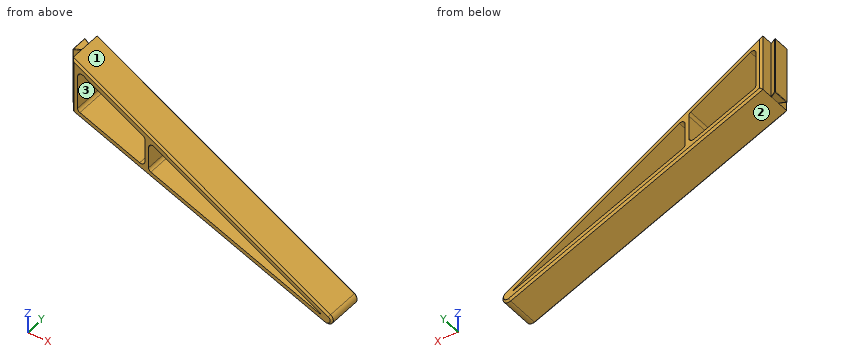
```python
from build123d import *

# Parameters (mm, degrees)
F1_DEPTH = 20
F3_DEPTH = 30
F4_R     = 2
F5_SIZE  = 1
F6_R     = 0.25


with BuildPart() as f1:
    # F0 (on Front) → F1 (new body)
    with BuildSketch(Plane.XZ):
        with BuildLine():
            Line((-46, 30), (-46, 0))
            Line((-46, 0), (89.051266, -55.940066))
            ThreePointArc((89.051266, -55.940066), (92.886071, -54.503098), (91.714375, -50.579104))
            Line((91.714375, -50.579104), (-46, 30))
        make_face()
        Polygon((-5, 2.534367), (90.199316, -53.168427), (-5, -13.735579), (-7, -12.907152), (-43, 2.004536), (-43, 24.768836), (-7, 3.704603), align=None, mode=Mode.SUBTRACT)
        Polygon((-5, -13.735579), (-5, 2.534367), (-7, 3.704603), (-7, -12.907152), align=None)
    extrude(amount=F1_DEPTH)

    # F2 (on Top) → F3 (join)
    with BuildSketch(Plane.XY):
        Polygon((-49.464102, -14.75), (-46, -12.75), (-46, -7.25), (-49.464102, -5.25), align=None)
    extrude(amount=F3_DEPTH)

    # F4
    f4_edges = [f1.edges().sort_by_distance(p)[0] for p in [
        (-7, -10, -12.907152),
        (-43, -10, 2.004536),
        (-43, -10, 24.768836),
        (-7, -10, 3.704603),
        (-5, -10, 2.534367),
        (-5, -10, -13.735579),
    ]]
    fillet(f4_edges, radius=F4_R)

    # F5
    f5_edges = [f1.edges().sort_by_distance(p)[0] for p in [
        (-46, 0, 15),
        (-46, -20, 15),
        (21.525633, -20, -27.970033),
        (21.525633, 0, -27.970033),
    ]]
    chamfer(f5_edges, length=F5_SIZE)

    # F6
    f6_edges = [f1.edges().sort_by_distance(p)[0] for p in [
        (-49.464102, -14.75, 15),
        (-49.464102, -5.25, 15),
        (-49.464102, -10, 0),
        (-49.464102, -10, 30),
        (-47.732051, -13.75, 30),
        (-47.732051, -6.25, 30),
        (-47.732051, -6.25, 0),
        (-47.732051, -13.75, 0),
        (90.199316, -10, -53.168427),
    ]]
    fillet(f6_edges, radius=F6_R)


solid = f1.part
```
Design review of the part built by this model. Coordinates are the model's own, in mm. Face numbers are marked on the shaded views. Coordinates: 2 decimals unless noted, no trailing zeros. Order: outer loops, then holes, each group sorted by start corner. A loop starts at its lowest first (then second) coordinate and runs counter-clockwise, first axis right, second up.
1) Mouldability with a two-part tool opening along Z and no side actions: class the marked faces 1, 2 and 3 as +Z half, -Z half, draft (parallel to the pull), parting line (faces both ways), or undercut.
2) Take a section at D-D, the plane y = -9.5. Give the boundary of the cut face in (x, z).
3) Wall thickness on line 1 along X through (y, z) = (-10.25, -1); line 2 along X through (y, z) = (-4, -24); line 3 along X through (y, z) = (-14.75, -16): over which ranges is each line inside the solid? List them lowest first.
4) Clearance check with flat-ended pins moving along their axes: pin 1 (8 mm diameter, centred on x = 66, y = -11.5, fed in from -Z); pin 2 (10 mm diameter, centred on y = -14, z = -21.5, fed in from -X); pin 3 (4 mm diameter, centred on x = 16.5, y = -13, fed in from -Z); pin 4 (12 mm diameter, centred on x = -28.5, z = -8.5, fed in from +Y). State where each tip first meets the part, or that it passes through.
5) Take a section at B-B, the plane z = -46. Give the boundary of the cut face in (x, y).
6) Take a section at A-A, the plane y = -16.75. Give the boundary of the cut face in (x, z).
7) Take a section at C-C, the plane x = 41.5. Give the boundary of the cut face in (y, z), and give its area (3 significant figures).
Returned:
1. face 1: +Z half
1. face 2: -Z half
1. face 3: undercut
2. outline: (-49.46, 0.25) arc R0.25 ccw to (-49.21, 0) - (-46, 0) - (89.05, -55.94) arc R3 ccw to (91.71, -50.58) - (-46, 30) - (-49.21, 30) arc R0.25 ccw to (-49.46, 29.75) - close; hole (-43, 3.34) arc R2 ccw to (-41.77, 1.49) - (-9.77, -11.76) arc R2 ccw to (-7, -9.91) - (-7, 2.56) arc R2 ccw to (-7.99, 4.28) - (-39.99, 23.01) arc R2 ccw to (-43, 21.28) - close; hole (-5, -12.4) arc R2 ccw to (-3.77, -14.25) - (86.83, -51.77) arc R0.25 ccw to (87.05, -51.32) - (-1.99, 0.77) arc R2 ccw to (-5, -0.95) - close
3. line 1: x = -43.59 to -35.75, -7 to -5, 1.04 to 6.98
3. line 2: x = 11.94 to 19.78, 40.35 to 46.29
3. line 3: x = -7.37 to 0.47, 26.68 to 32.62
4. pin 1: stops at z = -48.05
4. pin 2: stops at x = -6.17
4. pin 3: stops at z = -26.72
4. pin 4: stops at y = 0
5. outline: (65.05, -19) - (67.67, -20) - (72.89, -20) - (72.89, 0) - (67.67, 0) - (65.05, -1) - close; (77.95, -20) - (81.91, -20) - (83.89, -19) - (83.89, -1) - (81.91, 0) - (77.95, 0) - close
6. outline: (-46, 0) - (89.05, -55.94) arc R3 ccw to (91.71, -50.58) - (-46, 30) - close; hole (-43, 3.34) arc R2 ccw to (-41.77, 1.49) - (-9.77, -11.76) arc R2 ccw to (-7, -9.91) - (-7, 2.56) arc R2 ccw to (-7.99, 4.28) - (-39.99, 23.01) arc R2 ccw to (-43, 21.28) - close; hole (-5, -12.4) arc R2 ccw to (-3.77, -14.25) - (86.83, -51.77) arc R0.25 ccw to (87.05, -51.32) - (-1.99, 0.77) arc R2 ccw to (-5, -0.95) - close
7. outline: (-20, -35.16) - (-19, -36.24) - (-1, -36.24) - (0, -35.16) - (0, -33) - (-20, -33) - close; (-20, -24.67) - (0, -24.67) - (0, -22.36) - (-1, -21.2) - (-19, -21.2) - (-20, -22.36) - close
7. area: 132 mm2
